Here's how the part is built. I have some questions about the finished solid (model axes, mm). A direction names the side the tool comes from. Coordinates: 2 decimals unless noted, no trailing zeros. Loops run counter-clockwise (first coordinate to the right, second up) from the corner with the lowest first, then second, coordinate; pieces in that order, holes last. Notation, with made-up numbers: (52.5, 50) - (88.5, 50) arc R26 cw to (88.5, 67) - close; hole circle Ø11 at (-27.5, -33.75). An arc over 180 degrees is marked (long way). Use a Markdown table: item, result.
```python
from build123d import *

# Parameters (mm, degrees)
SKETCH_W             = 47.4
SKETCH_H             = 2
PAD_DEPTH            = 10
SKETCH002_W          = 15.5
SKETCH002_H          = 10
PAD001_DEPTH         = 1.5
SKETCH003_R          = 1.65
POCKET_DEPTH         = 2.001
POCKET_DEPTH_BACK    = 1.501
POCKET001_DEPTH      = 2.001
POCKET001_DEPTH_BACK = 1.501
SKETCH005_W          = 10
SKETCH005_H          = 10
PAD002_DEPTH         = 2.75


with BuildPart() as part:
    # Sketch → Pad (new body)
    with BuildSketch(Plane.XY):
        with Locations((0, 1)):
            Rectangle(SKETCH_W, SKETCH_H)
    extrude(amount=-PAD_DEPTH)

    # Sketch002 → Pad001 (join)
    with BuildSketch(Plane.XZ):
        with Locations((5.6, -5)):
            Rectangle(SKETCH002_W, SKETCH002_H)
    extrude(amount=PAD001_DEPTH)

    # Sketch003 → Pocket (cut, two sides)
    with BuildSketch(Plane.XZ) as pocket_sk:
        with Locations((-15.5, -5)):
            Circle(SKETCH003_R)
        with Locations((15.5, -5)):
            Circle(SKETCH003_R)
    extrude(amount=-POCKET_DEPTH, mode=Mode.SUBTRACT)
    extrude(pocket_sk.sketch, amount=POCKET_DEPTH_BACK, mode=Mode.SUBTRACT)

    # Sketch004 → Pocket001 (cut, two sides)
    with BuildSketch(Plane.XZ) as pocket001_sk:
        Polygon((-20.2, 0), (-23.7, -3.5), (-23.7, 0), align=None)
        Polygon((20.2, 0), (23.7, 0), (23.7, -3.5), align=None)
    extrude(amount=-POCKET001_DEPTH, mode=Mode.SUBTRACT)
    extrude(pocket001_sk.sketch, amount=POCKET001_DEPTH_BACK, mode=Mode.SUBTRACT)

    # Sketch005 → Pad002 (join)
    with BuildSketch(Plane.XZ):
        with Locations((-8.35, -5)):
            Rectangle(SKETCH005_W, SKETCH005_H)
    extrude(amount=PAD002_DEPTH)


solid = part.part
```
Q1. I want a section at C-C, the plane y = -0.9. Write out the boundary of the cut face in (x, z), then the cut area to 3 significant figures.
Check values:
| item | result |
|---|---|
| outline | (-13.35, -10) - (-3.35, -10) - (-3.35, 0) - (-13.35, 0) - close; (-2.15, -10) - (13.35, -10) - (13.35, 0) - (-2.15, 0) - close |
| area | 255 mm^2 |
Q2. I want a section at B-B, the plane x = 15.5. Write out the boundary of the cut face in (y, z).
Check values:
| item | result |
|---|---|
| outline | (0, -10) - (2, -10) - (2, -6.65) - (0, -6.65) - close; (0, -3.35) - (2, -3.35) - (2, 0) - (0, 0) - close |
Q3. If we mould it in two halves opening along X, with no side actions, what happens to faces 4 (the face through (13.35, -1, -5)), 5 (the face through (17.074, 0.986, -4.504)), 6 (the face through (-13.35, -1, -5))? For each: pulls with the +X half, pulls with the -X half, needs draft (parallel to the pull), parting line crosses it, or undercut.
Check values:
| item | result |
|---|---|
| face 4 | pulls with the +X half |
| face 5 | undercut |
| face 6 | pulls with the -X half |
Q4. Will these pins go through, and if not, where does the flat tip stop? P1, Ø1, axis at x = -2.5, z = -3, coming from the -Y side; P2, Ø3, axis at x = -15.5, z = -5, coming from the -Y side; P3, Ø2, axis at x = 16, z = -4.5, coming from the -Y side; P4, Ø0.8, axis at y = -0.5, z = -5, coming from the +X side.
Check values:
| item | result |
|---|---|
| P1 | y = -1.5 |
| P2 | through |
| P3 | y = 0 |
| P4 | x = 13.35 |
Q5. I want a section at A-A, the plane z = -5. Write out the boundary of the cut face in (x, y).
Check values:
| item | result |
|---|---|
| outline | (-23.7, 0) - (-17.15, 0) - (-17.15, 2) - (-23.7, 2) - close; (-13.85, 0) - (-13.35, 0) - (-13.35, -2.75) - (-3.35, -2.75) - (-3.35, 0) - (-2.15, 0) - (-2.15, -1.5) - (13.35, -1.5) - (13.35, 0) - (13.85, 0) - (13.85, 2) - (-13.85, 2) - close; (17.15, 0) - (23.7, 0) - (23.7, 2) - (17.15, 2) - close |
Q6. I want a section at D-D, the plane y = 1.25. Write out the boundary of the cut face in (x, z), then the cut area to 3 significant figures.
Check values:
| item | result |
|---|---|
| outline | (-23.7, -10) - (23.7, -10) - (23.7, -3.5) - (20.2, 0) - (-20.2, 0) - (-23.7, -3.5) - close; hole circle Ø3.3 at (-15.5, -5); hole circle Ø3.3 at (15.5, -5) |
| area | 445 mm^2 |
Q7. Please list where these lines run through material, in increasing order: L1, parallel to X at y = -0.45, z = -2.5; L2, parallel to Y at x = 2, z = -1.25; L3, parallel to Z at x = -15.5, y = 1.65. Write a range as from..to.
Check values:
| item | result |
|---|---|
| L1 | -13.35..-3.35, -2.15..13.35 |
| L2 | -1.5..2 |
| L3 | -10..-6.65, -3.35..0 |
Q8. Which directions (+Z, -Z, +X, -X, +Y, -Y) give clear straight access to the entire face, cutting with the end or side of a thin tool? Please do faces 1 (the face through (-19, 0, -5)), 2 (the face through (-2.15, -1, -5)), 3 (the face through (18, 0, -5)).
Check values:
| item | result |
|---|---|
| face 1 | +Z, -Z, -X, -Y |
| face 2 | +Z, -Z, -Y |
| face 3 | +Z, -Z, +X, -Y |
